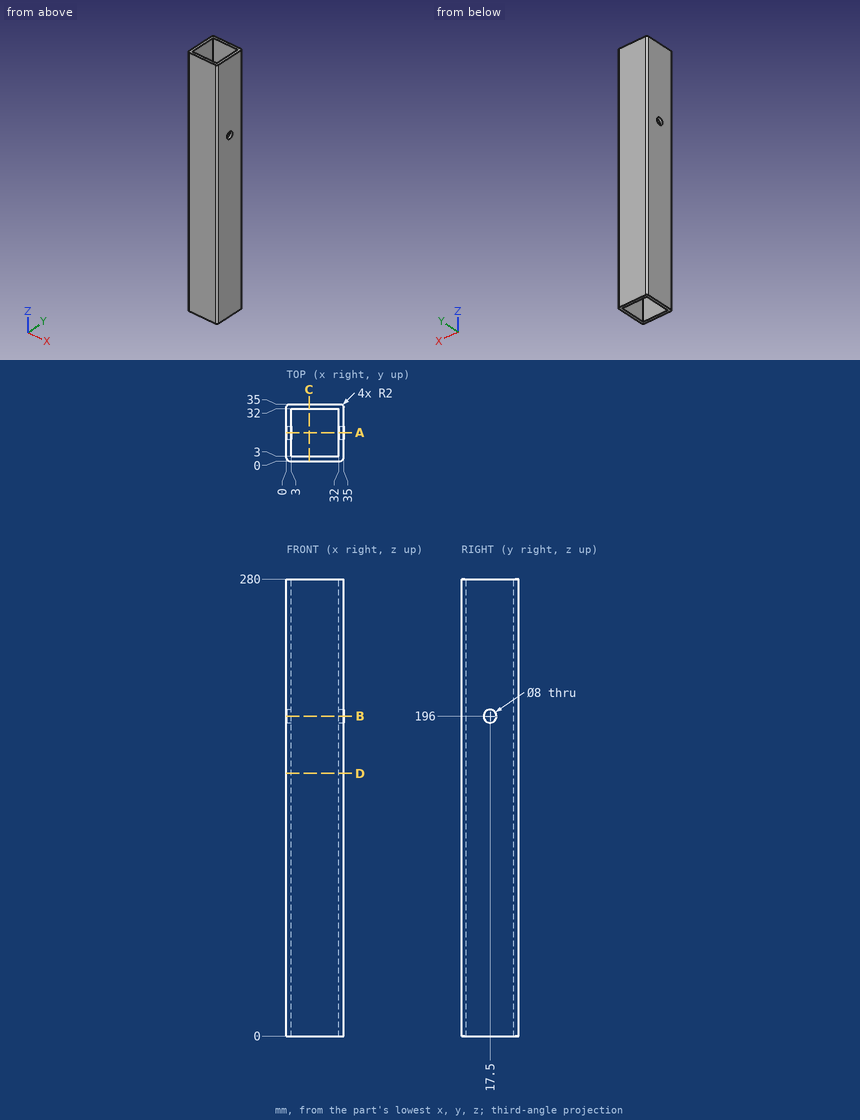
Print and shaded views of the part. All mm, measured from the part's lowest x, y and z. Coordinates: 2 decimals unless noted, no trailing zeros. Loops run counter-clockwise (first coordinate to the right, second up) from the corner with the lowest first, then second, coordinate; pieces in that order, holes last. Notation, with made-up numbers: (-37, 24.25) - (14, 24.25) arc R25 cw to (14, 59.25) - close; hole circle Ø7 at (34, 80). An arc over 180 degrees is marked (long way). Write item = value, one per line. Start each with the question number.
Item 1: Saw through at D-D, the plane z = 161. List the corners of the cut face in (x, y).
Item 2: Saw through at A-A, the plane y = 17.5. List the corners of the cut face in (x, z).
Item 3: Saw through at B-B, the plane z = 196. List the corners of the cut face in (x, y), then the cut area to 3 significant figures.
Item 4: Wall check: probe 1 along X at (y, z) = (31.5, 117); probe 2 along Y at (x, z) = (33.4, 196). Give the ranges that are in metal, low to high. Write a range as [from, to].
Item 5: Saw through at C-C, the plane x = 14. List the corners of the cut face in (y, z).
Answers:
q1.outline = (0, 2) arc R2 ccw to (2, 0) - (33, 0) arc R2 ccw to (35, 2) - (35, 33) arc R2 ccw to (33, 35) - (2, 35) arc R2 ccw to (0, 33) - close; hole (3, 3) - (32, 3) - (32, 32) - (3, 32) - close
q2.outline = (0, 0) - (3, 0) - (3, 192) - (0, 192) - close; (0, 200) - (3, 200) - (3, 280) - (0, 280) - close; (32, 0) - (35, 0) - (35, 192) - (32, 192) - close; (32, 200) - (35, 200) - (35, 280) - (32, 280) - close
q3.outline = (0, 2) arc R2 ccw to (2, 0) - (33, 0) arc R2 ccw to (35, 2) - (35, 13.5) - (32, 13.5) - (32, 3) - (3, 3) - (3, 13.5) - (0, 13.5) - close; (0, 21.5) - (3, 21.5) - (3, 32) - (32, 32) - (32, 21.5) - (35, 21.5) - (35, 33) arc R2 ccw to (33, 35) - (2, 35) arc R2 ccw to (0, 33) - close
q3.area = 333 mm2
q4.probe_1 = [0, 3], [32, 35]
q4.probe_2 = [0.04, 13.5], [21.5, 34.96]
q5.outline = (0, 0) - (3, 0) - (3, 280) - (0, 280) - close; (32, 0) - (35, 0) - (35, 280) - (32, 280) - close
